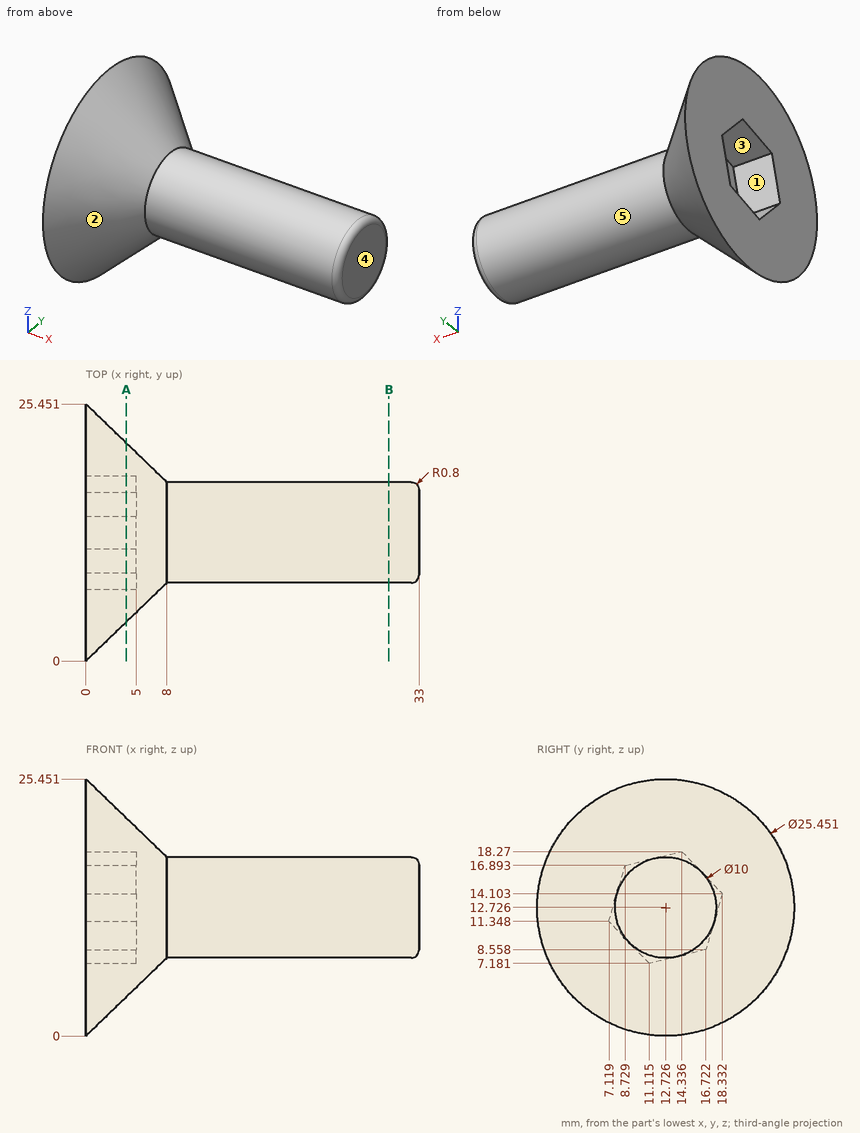
Design review of the part shown in the three views and the two pictorial views. Dimensions are in mm from the part's minimum x, y and z. A direction names the side the tool comes from. Round coordinates to 2 decimals unless told otherwise and drop trailing zeros. Write each loop counter-clockwise with the first axis right and the second up, starting at its lowest first coordinate (ties: lowest second). Pieces come first, ordered by that corner, then holes. Notation, with made-up numbers: (55, 71) -> (109, 71) arc R9 ccw to (109, 79) -> close; hole circle Ø5 at (25, 67). An arc over 180 degrees is marked (long way). Use one line per item in the form item = value.
1) Take a section at A-A, the plane x = 4. Write out the cut boundary in (y, z) (1 decimal).
Found:
outline = circle Ø17.7 at (12.7, 12.7); hole (7.1, 11.3) -> (11.1, 7.2) -> (16.7, 8.6) -> (18.3, 14.1) -> (14.3, 18.3) -> (8.7, 16.9) -> close
2) Clearance check with flat-ended pins moving along their axes: pin 1 (3.5 mm diameter, centred on y = 10, z = 14.5, fed in from -X); pin 2 (1 mm diameter, centred on x = 12, y = 12, fed in from +Z); pin 3 (10 mm diameter, centred on x = 26.5, z = 8.5, fed in from +Y) (1 decimal). State where each tip first meets the part, or that it passes through.
Found:
pin_1 = 5
pin_2 = 17.72
pin_3 = 17.7
3) Tool access review of the marked faces 1 and 2: name each direction out of +Z, -Z, +X, -X, +Y, -Y from which nothing blocks a thin tool from reaching the whole face with its end or side.
Found:
face_1 = -X
face_2 = +X
4) Take a section at B-B, the plane x = 30. Write out the cut boundary in (y, z) (1 decimal).
Found:
outline = circle Ø10 at (12.7, 12.7)
5) To check wall thickness, follow L1, parallel to Z at x = 17, y = 15.5 (1 decimal); L2, parallel to X at y = 21.75, z = 13.75 (1 decimal). State the ranges of each line that lie inside material, in increasing order. Write a range as from..to.
Found:
L1 = 8.6..16.9
L2 = 0..3.8
6) Mouldability with a two-part tool opening along Z and no side actions: class the marked faces 3, 4 and 5 as +Z half, -Z half, draft (parallel to the pull), parting line (faces both ways), or undercut.
Found:
face_3 = undercut
face_4 = draft
face_5 = parting line
